Input: part model. Units: mm. Frame: model coordinates. A direction names the side the tool comes from. Coordinates: 2 decimals unless noted, no trailing zeros. Order: outer loops, then holes, each group sorted by start corner. A loop starts at its lowest first (then second) coordinate and runs counter-clockwise, first axis right, second up. Notation, with made-up numbers: (8.5, 25.5) -> (50.5, 25.5) arc R23 ccw to (50.5, 60.5) -> close; hole circle Ø3 at (40, 50). An arc over 180 degrees is marked (long way). Write each question's results on one line, items separated by ' | '.
```python
from build123d import *
from build123d.topology import SkipClean

# Parameters (mm, degrees)
BOSS_EXTRUDE1_DEPTH      = 4
SKETCH2_R                = 3.05
CUT_EXTRUDE1_DEPTH       = 2
SKETCH3_R                = 1.5
CUT_EXTRUDE2_DEPTH       = 22.633307653
CUT_EXTRUDE4_START       = -1.2
CUT_EXTRUDE4_DEPTH       = 1.2
CUT_EXTRUDE6_DEPTH       = 1.5
CUT_EXTRUDE7_DEPTH       = 0.7
BOSS_EXTRUDE3_DEPTH      = 2
CUT_EXTRUDE12_START      = -2
CUT_EXTRUDE12_DEPTH      = 2
SKETCH6_R                = 2.5
CUT_EXTRUDE13_DEPTH      = 22.777052142
SKETCH17_W               = 0.35
SKETCH17_H               = 1.45
CUT_EXTRUDE14_DEPTH      = 1.9
BOSS_EXTRUDE5_DEPTH      = 1.9
CUT_EXTRUDE15_DEPTH      = 22.9089023
CUT_EXTRUDE15_DEPTH_BACK = 22.9089023
CUT_EXTRUDE16_DEPTH      = 22.890865675
CUT_EXTRUDE16_DEPTH_BACK = 22.890865675
CUT_EXTRUDE17_DEPTH      = 24.837994882
CUT_EXTRUDE17_DEPTH_BACK = 24.837994882
CHAMFER1_SIZE            = 1.75
CUT_EXTRUDE18_DEPTH      = 24.837994882
BOSS_EXTRUDE6_DEPTH      = 1.9
CHAMFER2_SIZE            = 0.5


with BuildPart() as part:
    # Sketch1 → Boss-Extrude1 (new body)
    with BuildSketch(Plane(origin=(0, 0, 0), x_dir=(1, 0, 0), z_dir=(0, 1, 0))):
        with BuildLine():
            Line((6.5, -20), (6.5, -4.663689527))
            ThreePointArc((6.5, -4.663689527), (7.615773106, -2.449489743), (8, 0))
            ThreePointArc((8, 0), (7.615773106, 2.449489743), (6.5, 4.663689527))
            ThreePointArc((6.5, 4.663689527), (0, 8), (-6.5, 4.663689527))
            ThreePointArc((-6.5, 4.663689527), (-7.615773106, 2.449489743), (-8, 0))
            ThreePointArc((-8, 0), (-7.615773106, -2.449489743), (-6.5, -4.663689527))
            Line((-6.5, -4.663689527), (-6.5, -20))
            Line((-6.5, -20), (6.5, -20))
        make_face()
    extrude(amount=BOSS_EXTRUDE1_DEPTH)

    # Sketch2 → Cut-Extrude1 (cut)
    with BuildSketch(Plane.XZ):
        with Locations(Location((0, 0, 0), (0, 0, 270))):
            Circle(SKETCH2_R)
    extrude(amount=-CUT_EXTRUDE1_DEPTH, mode=Mode.SUBTRACT)

    # Sketch3 → Cut-Extrude2 (cut, through all)
    with BuildSketch(Plane.XZ.offset(-2)):
        with Locations(Location((0, 0, 0), (0, 0, 270))):
            Circle(SKETCH3_R)
    extrude(amount=-CUT_EXTRUDE2_DEPTH, mode=Mode.SUBTRACT)

    # Sketch5 → Cut-Extrude4 (cut)
    with BuildSketch(Plane(origin=(0, 4, 0), x_dir=(1, 0, 0), z_dir=(0, 1, 0)).offset(CUT_EXTRUDE4_START)):
        with BuildLine():
            Line((5.75, 2.5), (2.5, 5.75))
            Line((2.5, 5.75), (0.75, 5.75))
            Line((0.75, 5.75), (0.75, 7.964766161))
            ThreePointArc((0.75, 7.964766161), (0, 8), (-0.75, 7.964766161))
            Line((-0.75, 7.964766161), (-0.75, 5.75))
            Line((-0.75, 5.75), (-2.5, 5.75))
            Line((-2.5, 5.75), (-5.75, 2.5))
            Line((-5.75, 2.5), (-5.75, -6.75))
            Line((-5.75, -6.75), (-4.4, -6.75))
            Line((-4.4, -6.75), (-4.4, -8.2))
            Line((-4.4, -8.2), (-5.66, -10))
            Line((-5.66, -10), (-6.5, -10))
            Line((-6.5, -10), (-6.5, -11.2))
            Line((-6.5, -11.2), (-6.5, -15))
            Line((-6.5, -15), (6.5, -15))
            Line((6.5, -15), (6.5, -11.2))
            Line((6.5, -11.2), (6.5, -10))
            Line((6.5, -10), (6.5, -8.2))
            Line((6.5, -8.2), (4.4, -8.2))
            Line((4.4, -8.2), (4.4, -6.75))
            Line((4.4, -6.75), (5.75, -6.75))
            Line((5.75, -6.75), (5.75, 2.5))
        make_face()
    extrude(amount=CUT_EXTRUDE4_DEPTH, mode=Mode.SUBTRACT)

    # Sketch7 → Cut-Extrude6 (cut)
    with BuildSketch(Plane(origin=(0, 2.8, 0), x_dir=(1, 0, 0), z_dir=(0, 1, 0))):
        with BuildLine():
            Line((-4.999999999, -5.5), (-4.999999999, -6.75))
            Line((-4.999999999, -6.75), (-3.499999999, -6.75))
            Line((-3.499999999, -6.75), (-3.499999999, -5.5))
            ThreePointArc((-3.499999999, -5.5), (-4.249999999, -4.75), (-4.999999999, -5.5))
        make_face()
        with BuildLine():
            Line((3.500000001, -5.5), (3.500000001, -6.75))
            Line((3.500000001, -6.75), (5.000000001, -6.75))
            Line((5.000000001, -6.75), (5.000000001, -5.5))
            ThreePointArc((5.000000001, -5.5), (4.250000001, -4.75), (3.500000001, -5.5))
        make_face()
    extrude(amount=-CUT_EXTRUDE6_DEPTH, mode=Mode.SUBTRACT)

    # Sketch9 → Cut-Extrude7 (cut)
    with BuildSketch(Plane(origin=(0, 2.8, 0), x_dir=(1, 0, 0), z_dir=(0, 1, 0))):
        Polygon((-6.5, -15), (6.5, -15), (6.5, -11.2), (6.5, -10), (6.5, -8.2), (4.75, -8.2), (4.75, -6.2), (4.4, -6.2), (-4.4, -6.2), (-4.75, -6.2), (-4.75, -8.7), (-5.66, -10), (-6.5, -10), (-6.5, -11.2), align=None)
    extrude(amount=-CUT_EXTRUDE7_DEPTH, mode=Mode.SUBTRACT)

    # Sketch14 → Boss-Extrude3 (add)
    with SkipClean():  # the faces are left unmerged after this step: merging them gives an invalid solid
        with BuildSketch(Plane(origin=(0, 4, 0), x_dir=(1, 0, 0), z_dir=(0, 1, 0))):
            with BuildLine():
                Line((6.5, -4.663689527), (6.5, 2.5))
                Line((6.5, 2.5), (7.599342077, 2.5))
                ThreePointArc((7.599342077, 2.5), (7.907431546, -1.213476964), (6.5, -4.663689527))
            make_face()
            with BuildLine():
                Line((-6.5, -4.663689527), (-6.5, 2.5))
                Line((-6.5, 2.5), (-7.599342077, 2.5))
                ThreePointArc((-7.599342077, 2.5), (-7.907431546, -1.213476964), (-6.5, -4.663689527))
            make_face()
        extrude(amount=BOSS_EXTRUDE3_DEPTH)

    # Sketch15 → Cut-Extrude12 (cut)
    with SkipClean():  # the faces are left unmerged after this step: merging them gives an invalid solid
        with BuildSketch(Plane(origin=(0, 4, 0), x_dir=(1, 0, 0), z_dir=(0, 1, 0)).offset(CUT_EXTRUDE12_START)):
            with BuildLine():
                Line((2.5, 5.75), (-2.5, 5.75))
                Line((-2.5, 5.75), (-4.125, 4.125))
                Line((-4.125, 4.125), (-5.656854249, 5.656854249))
                ThreePointArc((-5.656854249, 5.656854249), (0, 8), (5.656854249, 5.656854249))
                Line((5.656854249, 5.656854249), (4.125, 4.125))
                Line((4.125, 4.125), (2.5, 5.75))
            make_face()
        extrude(amount=CUT_EXTRUDE12_DEPTH, mode=Mode.SUBTRACT)

    # Sketch6 → Cut-Extrude13 (cut, through all)
    with SkipClean():  # the faces are left unmerged after this step: merging them gives an invalid solid
        with BuildSketch(Plane(origin=(0, 2.8, 0), x_dir=(1, 0, 0), z_dir=(0, 1, 0))):
            with Locations(Location((0, 0, 0), (0, 0, 270))):
                Circle(SKETCH6_R)
        extrude(amount=-CUT_EXTRUDE13_DEPTH, mode=Mode.SUBTRACT)

    # Sketch17 → Cut-Extrude14 (cut)
    with SkipClean():  # the faces are left unmerged after this step: merging them gives an invalid solid
        with BuildSketch(Plane(origin=(0, 4, 0), x_dir=(1, 0, 0), z_dir=(0, 1, 0))):
            Polygon((-4.75, -6.75), (-4.4, -6.75), (-4.4, -8.2), (-4.75, -8.7), align=None)
            with Locations((4.575, -7.475)):
                Rectangle(SKETCH17_W, SKETCH17_H)
        extrude(amount=-CUT_EXTRUDE14_DEPTH, mode=Mode.SUBTRACT)

    # Sketch18 → Boss-Extrude5 (add)
    with SkipClean():  # the faces are left unmerged after this step: merging them gives an invalid solid
        with BuildSketch(Plane(origin=(0, 2.1, 0), x_dir=(1, 0, 0), z_dir=(0, 1, 0))):
            Polygon((-6.5, -10), (-6.5, -15), (-4.75, -15), (-4.75, -8.7), (-5.66, -10), align=None)
        extrude(amount=BOSS_EXTRUDE5_DEPTH)

    # Sketch19 → Cut-Extrude15 (cut, two sides: drawn at the far end of the back side and taken through both)
    with SkipClean():  # the faces are left unmerged after this step: merging them gives an invalid solid
        with BuildSketch(Plane(origin=(0, 4, 0), x_dir=(1, 0, 0), z_dir=(0, 1, 0)).offset(-CUT_EXTRUDE15_DEPTH_BACK)):
            Polygon((-6.5, -20), (-3.5, -20), (-3.5, -15), (-4.75, -15), (-4.75, -8.2), (-6.5, -8.2), align=None)
            Polygon((4.75, -8.2), (6.5, -8.2), (6.5, -20), (3.5, -20), (3.5, -15), (4.75, -15), align=None)
        extrude(amount=CUT_EXTRUDE15_DEPTH + CUT_EXTRUDE15_DEPTH_BACK, mode=Mode.SUBTRACT)

    # Sketch20 → Cut-Extrude16 (cut, two sides: drawn at the far end of the back side and taken through both)
    with SkipClean():  # the faces are left unmerged after this step: merging them gives an invalid solid
        with BuildSketch(Plane(origin=(0, 2.1, 0), x_dir=(1, 0, 0), z_dir=(0, 1, 0)).offset(-CUT_EXTRUDE16_DEPTH_BACK)):
            Polygon((4.75, -15), (1.75, -15), (4.75, -12), align=None)
            Polygon((-4.75, -15), (-1.75, -15), (-4.75, -12), align=None)
        extrude(amount=CUT_EXTRUDE16_DEPTH + CUT_EXTRUDE16_DEPTH_BACK, mode=Mode.SUBTRACT)

    # Sketch21 → Cut-Extrude17 (cut, two sides: drawn at the far end of the back side and taken through both)
    with SkipClean():  # the faces are left unmerged after this step: merging them gives an invalid solid
        with BuildSketch(Plane(origin=(3.5, 0, 0), x_dir=(0, 0, -1), z_dir=(1, 0, 0)).offset(-CUT_EXTRUDE17_DEPTH_BACK)):
            with BuildLine():
                Line((-18.75, 4), (-16.25, 4))
                ThreePointArc((-16.25, 4), (-17.5, 2.75), (-18.75, 4))
            make_face()
        extrude(amount=CUT_EXTRUDE17_DEPTH + CUT_EXTRUDE17_DEPTH_BACK, mode=Mode.SUBTRACT)

    # Chamfer1
    # the kernel refuses this chamfer: 1.75 mm, written as the material it adds along each edge
    with BuildSketch(Plane(origin=(4.75, 0, 8.2), x_dir=(0.9996219169112968, 0, -0.027495876610586112), z_dir=(0, 1, 0))) as chamfer1_piece_1:
        Polygon((CHAMFER1_SIZE * 0.999621916911, -CHAMFER1_SIZE * 0.0274958766106), (-CHAMFER1_SIZE * 0.0274958766106, -CHAMFER1_SIZE * 0.999621916911), (0, 0), align=None)
    extrude(amount=2.1)
    with BuildSketch(Plane(origin=(-4.75, 2.1, 8.2), x_dir=(0.02749587661058662, 0, 0.9996219169112968), z_dir=(0, -1, 0))) as chamfer1_piece_2:
        Polygon((CHAMFER1_SIZE * 0.999621916911, CHAMFER1_SIZE * 0.0274958766106), (-CHAMFER1_SIZE * 0.0274958766106, CHAMFER1_SIZE * 0.999621916911), (0, 0), align=None)
    extrude(amount=2.1)

    # Sketch22 → Cut-Extrude18 (cut, through all)
    with BuildSketch(Plane(origin=(3.5, 0, 0), x_dir=(0, 0, -1), z_dir=(1, 0, 0))):
        with BuildLine():
            Line((-20, 0), (-17.5, 0))
            Line((-17.5, 0), (-17.5, 2.75))
            ThreePointArc((-17.5, 2.75), (-18.383883476, 3.116116524), (-18.75, 4))
            Line((-18.75, 4), (-20, 4))
            Line((-20, 4), (-20, 2.75))
            Line((-20, 2.75), (-20, 0))
        make_face()
    extrude(amount=-CUT_EXTRUDE18_DEPTH, mode=Mode.SUBTRACT)

    # Sketch24 → Boss-Extrude6 (add)
    with BuildSketch(Plane(origin=(0, 2.1, 0), x_dir=(1, 0, 0), z_dir=(0, 1, 0))):
        Polygon((-6.5, -8.2), (-4.75, -8.2), (-4.75, -9.95), align=None)
    extrude(amount=BOSS_EXTRUDE6_DEPTH)

    # Chamfer2
    chamfer2_edges = [part.edges().sort_by_distance(p)[0] for p in [
        (0, 0, 3.05),
    ]]
    chamfer(chamfer2_edges, length=CHAMFER2_SIZE)


solid = part.part
```
(1) Mould query, pull axis X, two halves, no side actions, for faces 5 (the face through (-3.23, 1.04, 13.52)), 6 (the face through (-7, 5, -2.5)), 7 (the face through (3.5, 2, 6)). Classes: +X half, -X half, draft (parallel to the pull), parting line (faces both ways), or undercut.
Return value:
face 5: -X half | face 6: draft | face 7: undercut
(2) Cut plane B-B, the plane y = 0.95. Return loops of the section in (x, z).
Return value:
outline: (-6.5, 4.66) arc R8 ccw (long way) to (6.5, 4.66) -> (6.5, 8.2) -> (4.75, 9.95) -> (4.75, 12) -> (1.75, 15) -> (3.5, 15) -> (3.5, 17.5) -> (-3.5, 17.5) -> (-3.5, 15) -> (-1.75, 15) -> (-4.75, 12) -> (-4.75, 9.95) -> (-6.5, 8.2) -> close; hole circle Ø6.1 at (0, 0)
(3) Cut plane C-C, the plane y = 5.3. Return loops of the section in (x, z).
Return value:
outline: (-7.6, -2.5) -> (-6.5, -2.5) -> (-6.5, 4.66) arc R8 ccw to start; (6.5, -2.5) -> (7.6, -2.5) arc R8 ccw to (6.5, 4.66) -> close
(4) Pin query (flat end, axial travel): P1, Ø1.8, axis at x = 5, y = 2.5, coming from the -Z side; P2, Ø1, axis at x = -5, y = 1.5, coming from the -Z side; P3, Ø1.1, axis at y = 1.5, z = 7.5, coming from the +X side; P4, Ø3, axis at x = -0.5, y = 1.5, coming from the -Z side. Return the tip coordinate at first contact, or that it passes through.
Return value:
P1: z = -6.78 | P2: z = -6.61 | P3: x = 6.5 | P4: z = -8
(5) Reachability of faces 1 (the face through (-4.93, 3.39, -3.32)), 2 (the face through (-7, 6, 0)), 3 (the face through (5, 3, -5)), 4 (the face through (6.5, 5, 1)) from +Z, -Z, +X, -X, +Y, -Y: full face, straight path, thin tool, end or side. Return the list, or none.
Return value:
face 1: +Y | face 2: +Z, -Z, +X, -X, +Y | face 3: -Z, +Y | face 4: +Z, -Z, +Y
(6) Line query: line 1 along Z through (x, y) = (-1.75, 2.3); line 2 along Y through (x, z) = (4, -2.5); line 3 along Y through (x, z) = (6, 5). Output: solid intervals per line, ascending. Write a range as from..to.
Return value:
line 1: -5.75..-1.79, 1.79..6.2, 15..17.5 | line 2: 0..2.8 | line 3: 0..4
(7) Cut plane A-A, the plane x = 0. Return loops of the section in (y, z), plus the area to 3 significant figures.
Return value:
outline: (0, -8) -> (2, -8) -> (2, -5.75) -> (2.8, -5.75) -> (2.8, -2.5) -> (2, -2.5) -> (2, -3.05) -> (0.5, -3.05) -> (0, -3.55) -> close; (0, 3.55) -> (0.5, 3.05) -> (2, 3.05) -> (2, 2.5) -> (2.8, 2.5) -> (2.8, 6.2) -> (2.1, 6.2) -> (2.1, 15) -> (4, 15) -> (4, 16.25) arc R1.25 cw to (2.75, 17.5) -> (0, 17.5) -> close | area: 48.8 mm2
(8) Cut plane D-D, the plane x = 6. Return loops of the section in (y, z).
Return value:
outline: (0, -5.29) -> (4, -5.29) -> (4, 8.2) -> (2.1, 8.2) -> (2.1, 8.7) -> (0, 8.7) -> close
